Source: CAD feature listing. Evaluate the final solid. Frame: model axes, mm. A direction names the side the tool comes from. Coordinates: 2 decimals unless noted, no trailing zeros. Write each loop counter-clockwise with the first axis right and the second up, starting at its lowest first coordinate (ties: lowest second). Pieces come first, ordered by that corner, then holes. Notation, with made-up numbers: (16.5, 64.5) -> (72.5, 64.5) arc R26 ccw to (72.5, 87.5) -> close; hole circle Ø11 at (-0.5, 82.5). An arc over 180 degrees is marked (long way). Write item = value, one per line.
from build123d import *

# Parameters (mm, degrees)
BOSS_EXTRUDE1_DEPTH = 127
SKETCH2_R           = 4.7625
CUT_EXTRUDE1_DEPTH  = 38.1


with BuildPart() as part:
    # Sketch1 → Boss-Extrude1 (new, symmetric)
    with BuildSketch(Plane.XY):
        with BuildLine():
            Line((-19.685, 25.4), (19.685, 25.4))
            ThreePointArc((19.685, 25.4), (23.726115254, 23.726115254), (25.4, 19.685))
            Line((25.4, 19.685), (25.4, -19.685))
            ThreePointArc((25.4, -19.685), (23.726115254, -23.726115254), (19.685, -25.4))
            Line((19.685, -25.4), (-19.685, -25.4))
            ThreePointArc((-19.685, -25.4), (-23.726115254, -23.726115254), (-25.4, -19.685))
            Line((-25.4, -19.685), (-25.4, 19.685))
            ThreePointArc((-25.4, 19.685), (-23.726115254, 23.726115254), (-19.685, 25.4))
        make_face()
        with BuildLine():
            Line((-19.685, -22.225), (19.685, -22.225))
            ThreePointArc((19.685, -22.225), (21.481051224, -21.481051224), (22.225, -19.685))
            Line((22.225, -19.685), (22.225, 19.685))
            ThreePointArc((22.225, 19.685), (21.481051224, 21.481051224), (19.685, 22.225))
            Line((19.685, 22.225), (-19.685, 22.225))
            ThreePointArc((-19.685, 22.225), (-21.481051224, 21.481051224), (-22.225, 19.685))
            Line((-22.225, 19.685), (-22.225, -19.685))
            ThreePointArc((-22.225, -19.685), (-21.481051224, -21.481051224), (-19.685, -22.225))
        make_face(mode=Mode.SUBTRACT)
    extrude(amount=BOSS_EXTRUDE1_DEPTH, both=True)

    # Sketch2 → Cut-Extrude1 (cut, symmetric)
    with BuildSketch(Plane(origin=(0, 0, 0), x_dir=(1, 0, 0), z_dir=(0, 1, 0))):
        with Locations(Location((0, 57.15, 0), (0, 0, 270))):
            Circle(SKETCH2_R)
        with Locations(Location((0, -57.15, 0), (0, 0, 270))):
            Circle(SKETCH2_R)
    extrude(amount=CUT_EXTRUDE1_DEPTH, both=True, mode=Mode.SUBTRACT)


solid = part.part
1) Cut plane B-B, the plane y = -2. Output: boundary loops of the cut face in (x, z) (3 decimals).
Answer block:
outline = (-25.4, -127) -> (-22.225, -127) -> (-22.225, 127) -> (-25.4, 127) -> close; (22.225, -127) -> (25.4, -127) -> (25.4, 127) -> (22.225, 127) -> close
2) Cut plane C-C, the plane x = 0. Output: boundary loops of the cut face in (y, z) (1 decimal), and give its area (3 significant figures).
Answer block:
outline = (-25.4, -127) -> (-22.2, -127) -> (-22.2, -61.9) -> (-25.4, -61.9) -> close; (-25.4, -52.4) -> (-22.2, -52.4) -> (-22.2, 52.4) -> (-25.4, 52.4) -> close; (-25.4, 61.9) -> (-22.2, 61.9) -> (-22.2, 127) -> (-25.4, 127) -> close; (22.2, -127) -> (25.4, -127) -> (25.4, -61.9) -> (22.2, -61.9) -> close; (22.2, -52.4) -> (25.4, -52.4) -> (25.4, 52.4) -> (22.2, 52.4) -> close; (22.2, 61.9) -> (25.4, 61.9) -> (25.4, 127) -> (22.2, 127) -> close
area = 1,490 mm2
3) Cut plane A-A, the plane z = -57.15. Output: boundary loops of the cut face in (x, y) (1 decimal), and give its area (3 significant figures).
Answer block:
outline = (-25.4, -19.7) arc R5.7 ccw to (-19.7, -25.4) -> (-4.8, -25.4) -> (-4.8, -22.2) -> (-19.7, -22.2) arc R2.5 cw to (-22.2, -19.7) -> (-22.2, 19.7) arc R2.5 cw to (-19.7, 22.2) -> (-4.8, 22.2) -> (-4.8, 25.4) -> (-19.7, 25.4) arc R5.7 ccw to (-25.4, 19.7) -> close; (4.8, -25.4) -> (19.7, -25.4) arc R5.7 ccw to (25.4, -19.7) -> (25.4, 19.7) arc R5.7 ccw to (19.7, 25.4) -> (4.8, 25.4) -> (4.8, 22.2) -> (19.7, 22.2) arc R2.5 cw to (22.2, 19.7) -> (22.2, -19.7) arc R2.5 cw to (19.7, -22.2) -> (4.8, -22.2) -> close
area = 522 mm2
4) First-contact query: pin 1 Ø11 at (x, z) = (0, -57.15) entering from +Y. Flat tip, straight axial feed; report the tip coordinate or a pass-through.
Answer block:
pin_1 = 25.4
5) Reachability of faces 1 (the cylindrical face through (-23.77, 23.68, 1.78)), 2 (the flat face through (0, -22.225, 2)) from +Z, -Z, +X, -X, +Y, -Y: full face, straight path, thin tool, end or side. Return the list, or none.
Answer block:
face_1 = +Z, -Z, -X, +Y
face_2 = +Z, -Z
6) Pull-direction query (Z, two-part tool) for faces 3 (the flat face through (0.1, -22.5, 127)), 4 (the cylindrical face through (0.209, 23.835, 52.392)), 5 (the cylindrical face through (23.77, -23.68, 1.78)); classes: +Z half, -Z half, draft (parallel to the pull), parting line (faces both ways), or undercut.
Answer block:
face_3 = +Z half
face_4 = undercut
face_5 = draft
7) Material intervals for probe 1 along Y at (x, z) = (2, 107) (3 decimals); probe 2 along X at (y, z) = (-23.4, 57.15), sorted ascending. Write a range as [from, to].
Answer block:
probe_1 = [-25.4, -22.225], [22.225, 25.4]
probe_2 = [-24.03, -4.76], [4.76, 24.03]
8) Cut plane D-D, the plane z = 45.5. Output: boundary loops of the cut face in (x, y) (3 decimals), and give its area (3 significant figures).
Answer block:
outline = (-25.4, -19.685) arc R5.715 ccw to (-19.685, -25.4) -> (19.685, -25.4) arc R5.715 ccw to (25.4, -19.685) -> (25.4, 19.685) arc R5.715 ccw to (19.685, 25.4) -> (-19.685, 25.4) arc R5.715 ccw to (-25.4, 19.685) -> close; hole (-22.225, -19.685) arc R2.54 ccw to (-19.685, -22.225) -> (19.685, -22.225) arc R2.54 ccw to (22.225, -19.685) -> (22.225, 19.685) arc R2.54 ccw to (19.685, 22.225) -> (-19.685, 22.225) arc R2.54 ccw to (-22.225, 19.685) -> close
area = 582 mm2
